Autodesk Fusion 360 part; units mm, degrees
sketch "스케치1" plane through (0, 0, 0) normal (0, 0, 1) x (1, 0, 0)
  line L0 (-36, 40) -> (36, 40)
  line L1 (40, 36) -> (40, -36)
  line L2 (36, -40) -> (-36, -40)
  line L3 (-40, -36) -> (-40, 36)
  line L4 (-30, 35) -> (30, 35)
  line L5 (35, 30) -> (35, -30)
  line L6 (30, -35) -> (-30, -35)
  line L7 (-35, -30) -> (-35, 30)
  arc A0 (-36, 40) -> (-40, 36) centre (-36, 36) ccw
  arc A1 (40, 36) -> (36, 40) centre (36, 36) ccw
  arc A2 (36, -40) -> (40, -36) centre (36, -36) ccw
  arc A3 (-40, -36) -> (-36, -40) centre (-36, -36) ccw
  arc A4 (-35, -30) -> (-30, -35) centre (-30, -30) ccw
  arc A5 (30, -35) -> (35, -30) centre (30, -30) ccw
  arc A6 (35, 30) -> (30, 35) centre (30, 30) ccw
  arc A7 (-30, 35) -> (-35, 30) centre (-30, 30) ccw
  line L8 (-35, -30) -> (-15.7004, -10.7004)
  line L9 (10.7004, 15.7004) -> (30, 35)
  line L10 (-30, -35) -> (-10.7004, -15.7004)
  line L11 (15.7004, 10.7004) -> (35, 30)
  line L12 (-35, 30) -> (-15.7004, 10.7004)
  line L13 (10.7004, -15.7004) -> (30, -35)
  line L14 (-30, 35) -> (-10.7004, 15.7004)
  line L15 (15.7004, -10.7004) -> (35, -30)
  circle A8 centre (0, 0) radius 14
  arc A9 (-10.7004, -15.7004) -> (10.7004, -15.7004) centre (0, 0) ccw
  arc A10 (15.7004, -10.7004) -> (15.7004, 10.7004) centre (0, 0) ccw
  arc A11 (10.7004, 15.7004) -> (-10.7004, 15.7004) centre (0, 0) ccw
  arc A12 (-15.7004, 10.7004) -> (-15.7004, -10.7004) centre (0, 0) ccw
  point P0 (-40, 40)
  point P1 (40, 40)
  point P2 (40, -40)
  point P3 (-35, 35)
  point P4 (35, -35)
  point P5 (-35, -35)
  dimension "d1" = 80
  dimension "d2" = 80
  dimension "d3" = 40
  dimension "d4" = 40
  dimension "d5" = 70
  dimension "d6" = 70
  dimension "d7" = 5
  dimension "d8" = 5
  dimension "d9" = 4
  dimension "d10" = 38
  dimension "d11" = 5
  dimension "d12" = 28
extrude "돌출1" add sketch "스케치1" along normal blind 5 contours L0 L1 L2 L3 A0 A1 A2 A3 | A4 A5 A6 A7 L8 L9 L10 L11 L12 L13 L14 L15 A9 A10 A11 A12
sketch "스케치2" plane through (0, 0, 5) normal (0, 0, 1) x (-1, 0, 0)
  circle A0 centre (35, 35) radius 1.7
  dimension "d15" = 3.4
extrude "돌출2" cut sketch "스케치2" against normal through all
sketch "스케치9" plane through (0, 0, 0) normal (0, 0, -1) x (1, 0, 0)
  line L0 (15.7004, -10.7004) -> (35, -30)
  arc A0 (36, -40) -> (40, -36) centre (36, -36) ccw construction
  line L1 (51.5725, -26.0844) -> (40, -14.5118) construction
  line L2 (40, -14.5118) -> (51.5725, -26.0844)
  line L3 (38.8284, -38.8284) -> (51.5725, -26.0844)
  line L4 (40, -14.5118) -> (38.8284, -38.8284)
  line L5 (38.8284, -38.8284) -> (26.0844, -51.5725)
  line L6 (14.5118, -40) -> (38.8284, -38.8284)
  line L7 (14.5118, -40) -> (26.0844, -51.5725)
  point P0 (-14.5118, 40)
  point P1 (-40, 14.5118)
extrude "돌출6" add sketch "스케치9" against normal blind 5
sketch "스케치10" plane through (38.8284, 38.8284, 0) normal (0.7071, 0.7071, 0) x (-0.7071, 0.7071, 0)
  circle A0 centre (-9.7, 2.5) radius 1.7
  line L0 (0, 0) -> (0, -7)
  circle A1 centre (9.7, 2.5) radius 1.7
  dimension "d46" = 3.4
  dimension "d47" = 9.7
extrude "돌출7" cut sketch "스케치10" against normal blind 2
sketch "스케치11" plane through (37.4142, 37.4142, 0) normal (0.7071, 0.7071, 0) x (-0.7071, 0.7071, 0)
  circle A0 centre (-9.7, 2.5) radius 1.25
  circle A1 centre (9.7, 2.5) radius 1.25
  point P0 (-9.7, 2.5)
  point P1 (9.7, 2.5)
  dimension "d50" = 2.5
  dimension "d51" = 2.5
extrude "돌출8" cut sketch "스케치11" against normal blind 2
fillet "모깎기1" radius 5 2 edges at (26.0844, 51.5725, 2.5) (51.5725, 26.0844, 2.5)
fillet "모깎기2" radius 28.5 2 edges at (40, 14.5118, 2.5) (14.5118, 40, 2.5)
Geometry check sheet. Reference: the model listing, model coordinates, mm. A direction names the side the tool comes from. Coordinates: 2 decimals unless noted, no trailing zeros. Order: outer loops, then holes, each group sorted by start corner. A loop starts at its lowest first (then second) coordinate and runs counter-clockwise, first axis right, second up. Notation, with made-up numbers: M 2.25,-17.75 L 17.25,-17.75 A23 cw 17.25,13.25 Z; hole C 54.25,-19.5 d1. An arc over 180 degrees is marked long. One line per question, with ' | ' between items. Start each with the question number.
Item 1: Gauge pin test, flat ends, axial feed: pin 1 (1.5 mm diameter, centred on y = -9.5, z = 1, fed in from +X); pin 2 (1.5 mm diameter, centred on x = 10.5, z = 3, fed in from +Y); pin 3 (1.5 mm diameter, centred on x = -13, z = 3.5, fed in from +Y); pin 4 (8 mm diameter, centred on x = -17.5, y = -27, fed in from +Z). Record the tip position at first contact, or that the pin passes through.
Item 2: Cross-section at A-A on x = 0. Enter the section's corners in (y, z).
Item 3: Draft check along Y on faces 3 (the flat face through (35, 0, 2)), 4 (the flat face through (-6, 15, 5)), 5 (the cylindrical face through (-38.797, -38.859, 2.465)), 6 (the flat face through (-17, 40, 2)). Enter one of: pulls with the +Y half, pulls with the -Y half, needs draft (parallel to the pull), parting line crosses it, or undercut.
Item 4: Set-up check for faces 1 (the cylindrical face through (0, -19, 2)), 2 (the cylindrical face through (-38.859, 38.797, 2.465)): record each of +Z, -Z, +X, -X, +Y, -Y from which the full face is reachable in a straight line by a thin tool's end or side.
Item 5: Material ranges on L1, parallel to X at y = 21, z = 4.15; L2, parallel to Y at x = -0.5, z = 1.25; L3, parallel to X at y = 22.5, z = 0.5, recorded low to high. Write a range as [from, to].
Findings:
1) pin 1: stops at x = 40 | pin 2: stops at y = 41.31 | pin 3: stops at y = 40 | pin 4: stops at z = 5
2) outline: M -40,0 L -35,0 L -35,5 L -40,5 Z; M -19,0 L -14,0 L -14,5 L -19,5 Z; M 14,0 L 19,0 L 19,5 L 14,5 Z; M 35,0 L 40,0 L 40,5 L 35,5 Z
3) face 3: undercut | face 4: needs draft | face 5: pulls with the -Y half | face 6: pulls with the +Y half
4) face 1: +Z, -Z | face 2: +Z, -Z, -X, +Y
5) L1: x = [-40, -35], [-26, -16], [16, 26], [35, 46.64] | L2: y = [-40, -35], [-18.99, -13.99], [13.99, 18.99], [35, 40] | L3: x = [-40, -35], [-27.5, -17.5], [17.5, 27.5], [35, 47.99]
